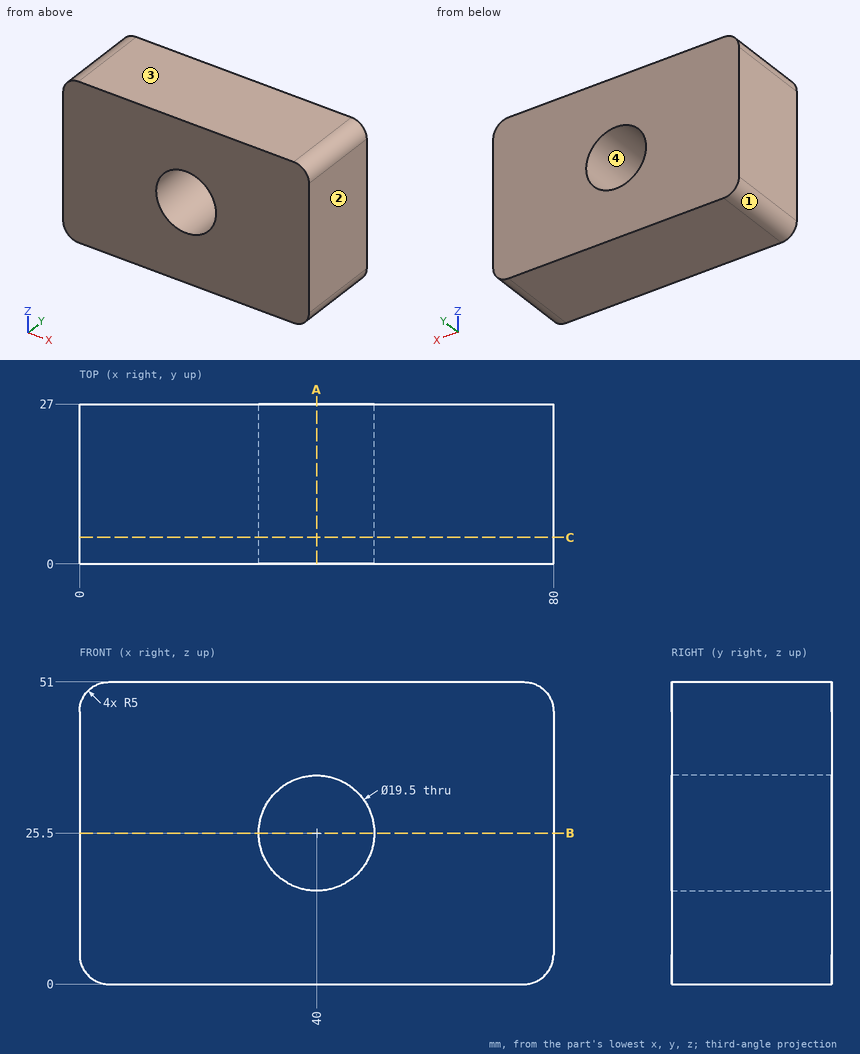
Input: dimensioned drawing with shaded views. Units: mm. Origin: part minimum x, y, z. Coordinates: 2 decimals unless noted, no trailing zeros. Order: outer loops, then holes, each group sorted by start corner. A loop starts at its lowest first (then second) coordinate and runs counter-clockwise, first axis right, second up. Notation, with made-up numbers: (-11.75, 66) - (3.25, 66) arc R21 cw to (3.25, 92) - close; hole circle Ø10 at (-28, -19). An arc over 180 degrees is marked (long way). Put each result on its own line as item: value.
1. Draft query along Z for the marked faces 1, 2, 3 and 4. Return one class per face: pulls with the +Z half, pulls with the -Z half, needs draft (parallel to the pull), parting line crosses it, or undercut.
Report:
face 1: pulls with the -Z half
face 2: needs draft
face 3: pulls with the +Z half
face 4: undercut
2. Cut plane C-C on y = 4.5. Return the cut outline in (x, z).
Report:
outline: (0, 5) arc R5 ccw to (5, 0) - (75, 0) arc R5 ccw to (80, 5) - (80, 46) arc R5 ccw to (75, 51) - (5, 51) arc R5 ccw to (0, 46) - close; hole circle Ø19.5 at (40, 25.5)
3. Line query: line 1 along X through (y, z) = (20.5, 25.5); line 2 along Z through (x, y) = (31.5, 1); line 3 along X through (y, z) = (14.25, 27.5). Output: solid intervals per line, ascending.
Report:
line 1: x = 0 to 30.25, 49.75 to 80
line 2: z = 0 to 20.72, 30.28 to 51
line 3: x = 0 to 30.46, 49.54 to 80
4. Cut plane B-B on z = 25.5. Return the cut outline in (x, y).
Report:
outline: (0, 0) - (30.25, 0) - (30.25, 27) - (0, 27) - close; (49.75, 0) - (80, 0) - (80, 27) - (49.75, 27) - close
5. Cut plane A-A on x = 40. Return the cut outline in (y, z).
Report:
outline: (0, 0) - (27, 0) - (27, 15.75) - (0, 15.75) - close; (0, 35.25) - (27, 35.25) - (27, 51) - (0, 51) - close
